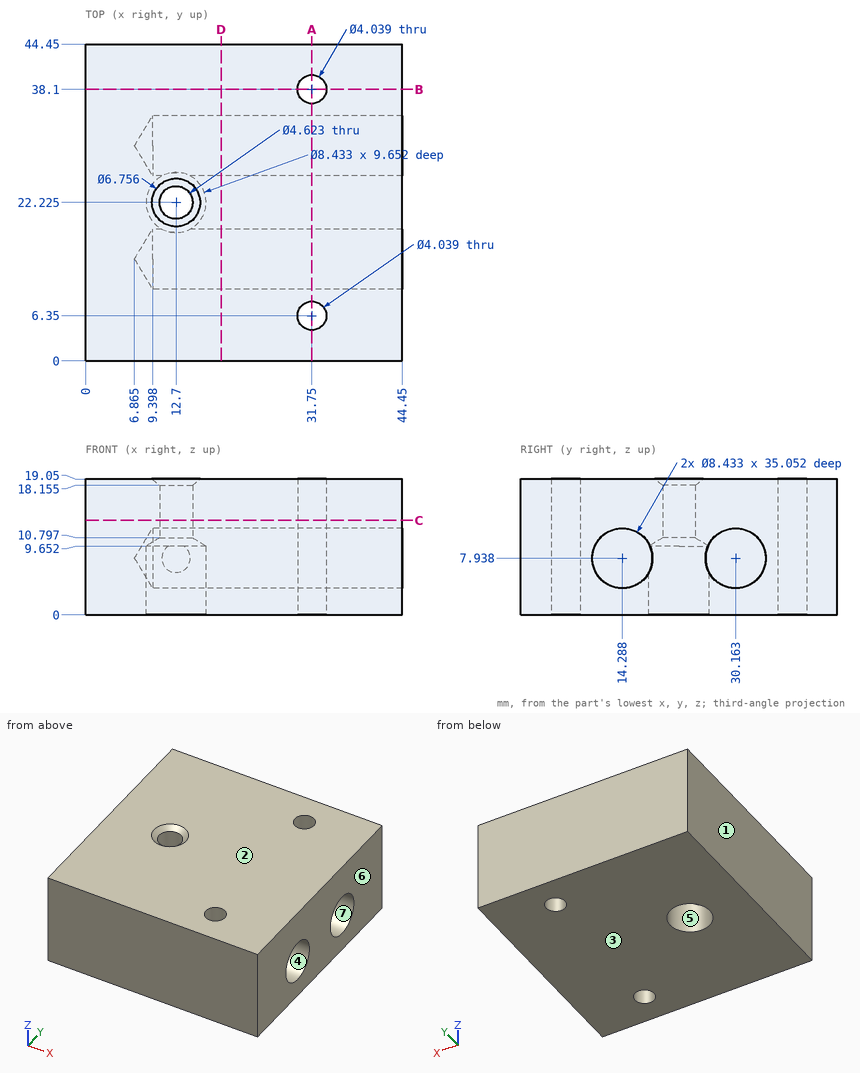
Job drawing, mm, ordinate dimensions from the low corner. One solid piece. A direction names the side the tool comes from. Coordinates: 2 decimals unless noted, no trailing zeros. Write each loop counter-clockwise with the first axis right and the second up, starting at its lowest first coordinate (ties: lowest second). Pieces come first, ordered by that corner, then holes. Notation, with made-up numbers: (-17, 76.25) - (25, 76.25) arc R16 ccw to (25, 84.25) - close; hole circle Ø5 at (62.5, 16). An arc over 180 degrees is marked (long way). Use a Markdown table: item, result. Add a question column.
Item 1: Band-saw the part on C-C, the plane z = 13.25. Give the number of separate pieces and of enclosed holes in the cut face, and give its area (3 significant figures).
Item 2: Mould opens along Z. For the marked faces 1, 2, 3 and 4 say: pulls with the +Z half, pulls with the -Z half, needs draft (parallel to the pull), parting line crosses it, or undercut.
Item 3: Band-saw the part on D-D, the plane x = 19. Give the cut face in (y, z), and give its area (3 significant figures).
Item 4: Band-saw the part on B-B, the plane y = 38.1. Give the cut face in (x, z).
Item 5: 3-axis set-ups, long thin cutter, end or side, ignore diameter. For the marked faces 5, 6 and 7: which of +Z, -Z, +X, -X, +Y, -Y reach the whole face in a straight line?
Item 6: Drill centre lines: L1, parallel to Y at x = 31.75, z = 8; L2, parallel to X at y = 23.5, z = 15.5; L3, parallel to X at y = 24, z = 12.25. Where is each one in solid material? Low to high. Write a range as from..to.
Item 7: Flat gauge pin, fed straight in: pin 1 (3 mm diameter, centred on x = 31.75, y = 38.1, fed in from +Z). Where does the tip first touch, or does it go through?
Item 8: Band-saw the part on A-A, the plane x = 31.75. Give the cut face in (y, z), and give its area (3 significant figures).
Numbers:
| question | item | result |
|---|---|---|
| 1 | separate pieces | 1 |
| 1 | enclosed holes | 3 |
| 1 | area | 1,930 mm2 |
| 2 | face 1 | needs draft |
| 2 | face 2 | pulls with the +Z half |
| 2 | face 3 | pulls with the -Z half |
| 2 | face 4 | undercut |
| 3 | outline | (0, 0) - (44.45, 0) - (44.45, 19.05) - (0, 19.05) - close; hole circle Ø8.43 at (14.29, 7.94); hole circle Ø8.43 at (30.16, 7.94) |
| 3 | area | 735 mm2 |
| 4 | outline | (0, 0) - (29.73, 0) - (29.73, 19.05) - (0, 19.05) - close; (33.77, 0) - (44.45, 0) - (44.45, 19.05) - (33.77, 19.05) - close |
| 5 | face 5 | -Z |
| 5 | face 6 | +Z, -Z, +X, +Y, -Y |
| 5 | face 7 | +X |
| 6 | L1 | 0..4.33, 8.37..10.07, 18.5..25.95, 34.38..36.08, 40.12..44.45 |
| 6 | L2 | 0..10.77, 14.63..44.45 |
| 6 | L3 | 0..11.22, 14.18..44.45 |
| 7 | pin 1 | through |
| 8 | outline | (0, 0) - (4.33, 0) - (4.33, 19.05) - (0, 19.05) - close; (8.37, 0) - (36.08, 0) - (36.08, 19.05) - (8.37, 19.05) - close; (40.12, 0) - (44.45, 0) - (44.45, 19.05) - (40.12, 19.05) - close; hole circle Ø8.43 at (14.29, 7.94); hole circle Ø8.43 at (30.16, 7.94) |
| 8 | area | 581 mm2 |
